Could you check a few things on this model? Use its own coordinates, in mm. Face numbers are marked on the shaded views. Round coordinates to 2 decimals unless told otherwise and drop trailing zeros. Write each loop counter-clockwise with the first axis right and the second up, starting at its lowest first coordinate (ties: lowest second). Pieces come first, ordered by that corner, then holes.
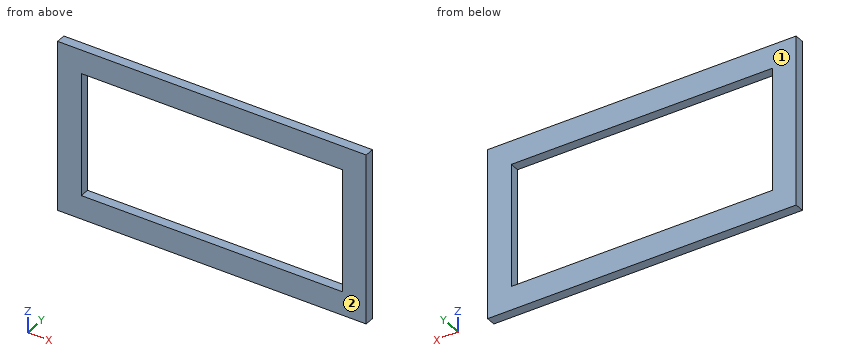
```python
from build123d import *

# Parameters (mm, degrees)
SKETCH1_W = 50
SKETCH1_H = 20


with BuildPart() as part:
    # Sweep1: sweep along a curve in space
    with BuildLine() as sweep1_path:
        Line((0, 0, 0), (650, 0, 0))
        Line((650, 0, 0), (650, 0, -360))
        Line((650, 0, -360), (0, 0, -360))
        Line((0, 0, -360), (0, 0, 0))
    # Sketch1 → Sweep1 (sweep)
    with BuildSketch(Plane(origin=(0, 0, 0), x_dir=(0, 0, -1), z_dir=(1, 0, 0))):
        with Locations((25, 10)):
            Rectangle(SKETCH1_W, SKETCH1_H)
    sweep(path=sweep1_path.line, transition=Transition.RIGHT)


solid = part.part
```
Q1. If I drill on L1, parallel to X at y = 3.25, z = -224; L2, parallel to Z at x = 284.5, y = 3.75, over which ranges is the centre line in solid material (lowest first)?
Q2. Imagine slicing it at A-A, the plane z = -216. Write out the boundary of the cut face in (x, y), then the cut area to 3 significant figures.
Q3. We'd pull the mould along Y, two halves only. Please class the marked faces 1 and 2: pulls with the +Y half, pulls with the -Y half, needs draft (parallel to the pull), parting line crosses it, or undercut.
Q4. Imagine slicing it at B-B, the plane y = 13. Write out the boundary of the cut face in (x, z).
Q5. Imagine slicing it at C-C, the plane x = 463. Write out the boundary of the cut face in (y, z).
Results found:
1. L1: x = 0 to 50, 600 to 650
1. L2: z = -360 to -310, -50 to 0
2. outline: (0, 0) - (50, 0) - (50, 20) - (0, 20) - close; (600, 0) - (650, 0) - (650, 20) - (600, 20) - close
2. area: 2,000 mm2
3. face 1: pulls with the +Y half
3. face 2: pulls with the -Y half
4. outline: (0, -360) - (650, -360) - (650, 0) - (0, 0) - close; hole (50, -310) - (600, -310) - (600, -50) - (50, -50) - close
5. outline: (0, -360) - (20, -360) - (20, -310) - (0, -310) - close; (0, -50) - (20, -50) - (20, 0) - (0, 0) - close
